Drawing for the job (mm, zero at the part's lowest x, y, z). Coordinates: 2 decimals unless noted, no trailing zeros. Loops run counter-clockwise (first coordinate to the right, second up) from the corner with the lowest first, then second, coordinate; pieces in that order, holes last. Notation, with made-up numbers: (47.5, -17) - (64.5, -17) arc R18 cw to (64.5, -12) - close; hole circle Ø2 at (-28.5, 14). An arc over 180 degrees is marked (long way). Put each result on its own line as item: value.
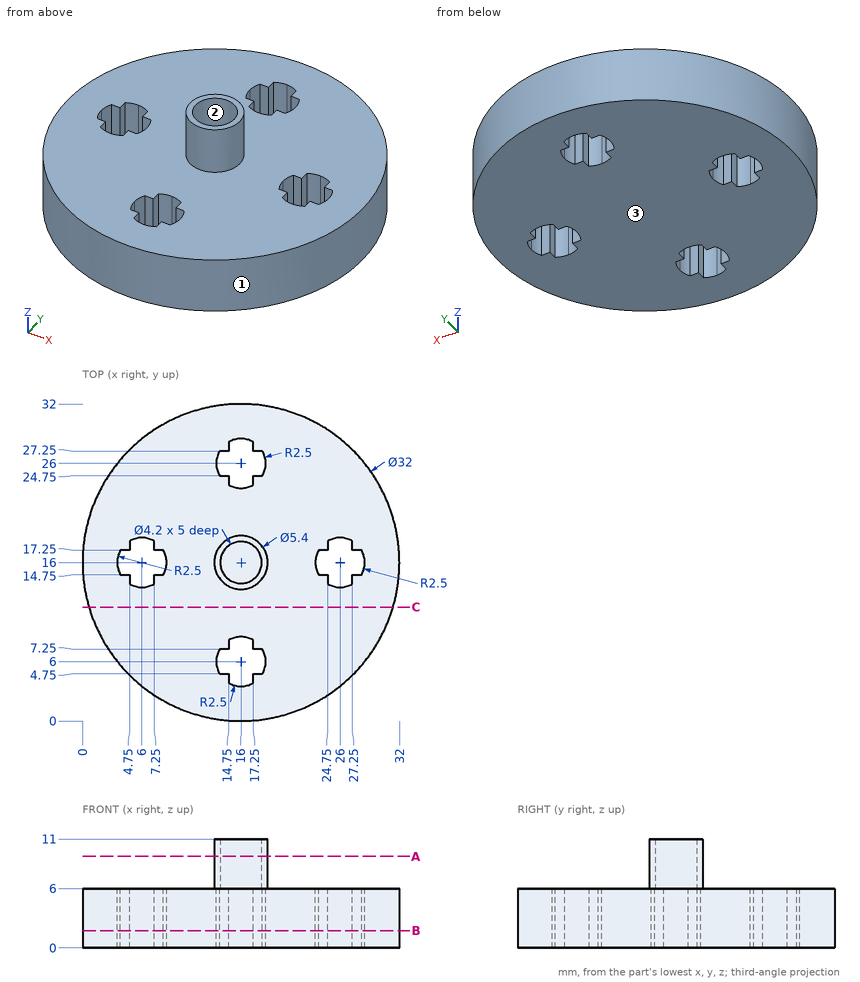
Q1. Pin check, flat tips, straight feed: pin 1 Ø1 at (x, y) = (18.5, 11) entering from -Z; pin 2 Ø1 at (x, z) = (7.5, 2) entering from +Y; pin 3 Ø1 at (x, z) = (17.5, 2.5) entering from +Y; pin 4 Ø1 at (x, z) = (8, 4.5) entering from -Y. Stop position of each tip, or through.
Determined:
pin 1: z = 0
pin 2: y = 29.86
pin 3: y = 31.97
pin 4: y = 1.87
Q2. Slice it at C-C, the plane y = 11.5. Give the cut face in (x, z), then the cut area to 3 significant figures.
Determined:
outline: (0.65, 0) - (31.35, 0) - (31.35, 6) - (0.65, 6) - close
area: 184 mm2
Q3. Slice it at B-B, the plane z = 1.75. State how many separate pieces and enclosed holes the cut face has, then the cut area to 3 significant figures.
Determined:
separate pieces: 1
enclosed holes: 4
area: 734 mm2
Q4. Wall check: L1, parallel to Y at x = 16, z = 8.3; L2, parallel to Z at x = 24, y = 18.5; L3, parallel to Y at x = 27, z = 3.25. Give the ranges that are in metal, low to high. Write a range as from..to.
Determined:
L1: 13.3..13.9, 18.1..18.7
L2: 0..6
L3: 4.38..13.71, 18.29..27.62
Q5. Slice it at A-A, the plane z = 9.25. Give the cut face in (x, y), then the cut area to 3 significant figures.
Determined:
outline: circle Ø5.4 at (16, 16); hole circle Ø4.2 at (16, 16)
area: 9.05 mm2
Q6. Mould opens along X. For the marked faces 1, 2 and 3 say: +X half, -X half, draft (parallel to the pull), parting line (faces both ways), or undercut.
Determined:
face 1: parting line
face 2: undercut
face 3: draft
